Source: CAD feature listing. Evaluate the final solid. Frame: model axes, mm. A direction names the side the tool comes from. Round coordinates to 2 decimals unless told otherwise and drop trailing zeros. Write each loop counter-clockwise with the first axis right and the second up, starting at its lowest first coordinate (ties: lowest second). Pieces come first, ordered by that corner, then holes.
from build123d import *

# Parameters (mm, degrees)
BOSS_EXTRUDE1_DEPTH = 19.05
FILLET1_R           = 15.875


with BuildPart() as part:
    # Sketch1 → Boss-Extrude1 (new body)
    with BuildSketch(Plane.XY):
        Polygon((0, 0), (47.625, -19.05), (79.375, -19.05), (133.35, 0), (133.35, -20.201691705), (82.638126498, -38.1), (43.956305212, -38.1), (0, -20.517477915), (-43.956305212, -38.1), (-82.638126498, -38.1), (-133.35, -20.201691705), (-133.35, 0), (-79.375, -19.05), (-47.625, -19.05), align=None)
    extrude(amount=BOSS_EXTRUDE1_DEPTH)

    # Fillet1
    fillet1_edges = [part.edges().sort_by_distance(p)[0] for p in [
        (0, 0, 9.525),
        (47.625, -19.05, 9.525),
        (79.375, -19.05, 9.525),
        (82.638126498, -38.1, 9.525),
        (43.956305212, -38.1, 9.525),
        (0, -20.517477915, 9.525),
        (-43.956305212, -38.1, 9.525),
        (-82.638126498, -38.1, 9.525),
        (-79.375, -19.05, 9.525),
        (-47.625, -19.05, 9.525),
    ]]
    fillet(fillet1_edges, radius=FILLET1_R)


solid = part.part
1) Section query C-C on z = 7.5. Return the cut outline in (x, y) (3 decimals).
Taken from the geometry:
outline: (-133.35, -20.202) - (-85.202, -37.195) arc R15.875 ccw to (-79.919, -38.1) - (-47.014, -38.1) arc R15.875 ccw to (-41.118, -36.965) - (-5.896, -22.876) arc R15.875 cw to (5.896, -22.876) - (41.118, -36.965) arc R15.875 ccw to (47.014, -38.1) - (79.919, -38.1) arc R15.875 ccw to (85.202, -37.195) - (133.35, -20.202) - (133.35, 0) - (81.939, -18.145) arc R15.875 cw to (76.656, -19.05) - (50.682, -19.05) arc R15.875 cw to (44.786, -17.915) - (5.896, -2.358) arc R15.875 ccw to (-5.896, -2.358) - (-44.786, -17.915) arc R15.875 cw to (-50.682, -19.05) - (-76.656, -19.05) arc R15.875 cw to (-81.939, -18.145) - (-133.35, 0) - close
2) Section query B-B on y = -33. Return the cut outline in (x, z), then the cut area to 3 significant figures.
Taken from the geometry:
outline: (-97.09, 0) - (-31.21, 0) - (-31.21, 19.05) - (-97.09, 19.05) - close; (31.21, 0) - (97.09, 0) - (97.09, 19.05) - (31.21, 19.05) - close
area: 2,510 mm2
3) Section query D-D on x = 73. Return the cut outline in (y, z), then the cut area to 3 significant figures.
Taken from the geometry:
outline: (-38.1, 0) - (-19.05, 0) - (-19.05, 19.05) - (-38.1, 19.05) - close
area: 363 mm2
4) Pull-direction query (X, two-part tool) for faces 4 (the face through (133.35, -10, 9)), 5 (the face through (-79.373, -18.816, 9.658)), 6 (the face through (-63, -38.1, 9)), 7 (the face through (-108.939, -28.817, 9.392)); classes: released by +X, released by -X, zero draft, split by the parting line, or undercut.
Taken from the geometry:
face 4: released by +X
face 5: undercut
face 6: zero draft
face 7: released by -X
5) Reachability of faces 1 (the face through (-25.613, -10.245, 9.392)), 2 (the face through (44.05, -37.82, 9.66)), 3 (the face through (2, -19, 0)) from +Z, -Z, +X, -X, +Y, -Y: full face, straight path, thin tool, end or side. Return the list, or none.
Taken from the geometry:
face 1: +Z, -Z, +Y
face 2: +Z, -Z, -Y
face 3: -Z, +X, -X, +Y, -Y
6) Contact query for flat-ended pins moving along their axis: P1, Ø1.5, axis at x = 105.5, z = 8.5, coming from the +Y side; P2, Ø4, axis at x = 1, z = 3.5, coming from the -Y side; P3, Ø5.5, axis at x = -60, z = 8, coming from the +Y side. Output: stop coordinate, or through.
Taken from the geometry:
P1: stops at y = -9.56
P2: stops at y = -22.03
P3: stops at y = -19.05
7) Material intervals for line 1 (Y direction, x = -52, z = 5); line 2 (Y direction, x = 112.5, z = 4.25), sorted ascending.
Taken from the geometry:
line 1: y = -38.1 to -19.05
line 2: y = -27.56 to -7.36
8) Section query A-A on y = -6. Return the cut outline in (x, z).
Taken from the geometry:
outline: (-133.35, 0) - (-116.35, 0) - (-116.35, 19.05) - (-133.35, 19.05) - close; (-15, 0) - (15, 0) - (15, 19.05) - (-15, 19.05) - close; (116.35, 0) - (133.35, 0) - (133.35, 19.05) - (116.35, 19.05) - close
